Geometry: final body of the model. Coordinates: model frame, mm. Face numbers are marked on the shaded views. A direction names the side the tool comes from. Round coordinates to 2 decimals unless told otherwise and drop trailing zeros. Loops run counter-clockwise (first coordinate to the right, second up) from the corner with the lowest first, then second, coordinate; pieces in that order, holes last. Notation, with made-up numbers: (77.5, -34) - (90.5, -34) arc R13 ccw to (90.5, -30) - close; hole circle Ø1 at (36, -35.75). An arc over 180 degrees is marked (long way). Use CSV: the item, a comma, the result in double quotes.
from build123d import *

# Parameters (mm, degrees)
BASE_EXTRUDE_DEPTH = 19.05


with BuildPart() as part:
    # Sketch1 → Base-Extrude (new body)
    with BuildSketch(Plane.XY):
        with BuildLine():
            Line((-76.2, -6.35), (-196.85, -6.35))
            ThreePointArc((-196.85, -6.35), (-199.09506403, -5.42006403), (-200.025, -3.175))
            Line((-200.025, -3.175), (-200.025, 41.275))
            ThreePointArc((-200.025, 41.275), (-199.09506403, 43.52006403), (-196.85, 44.45))
            Line((-196.85, 44.45), (-76.2, 44.45))
            ThreePointArc((-76.2, 44.45), (-73.95493597, 43.52006403), (-73.025, 41.275))
            Line((-73.025, 41.275), (-73.025, -3.175))
            ThreePointArc((-73.025, -3.175), (-73.95493597, -5.42006403), (-76.2, -6.35))
        make_face()
        with BuildLine():
            Line((-174.625, 11.1125), (-98.425, 11.1125))
            ThreePointArc((-98.425, 11.1125), (-90.4875, 19.05), (-98.425, 26.9875))
            Line((-98.425, 26.9875), (-174.625, 26.9875))
            ThreePointArc((-174.625, 26.9875), (-182.5625, 19.05), (-174.625, 11.1125))
        make_face(mode=Mode.SUBTRACT)
    extrude(amount=BASE_EXTRUDE_DEPTH)


solid = part.part
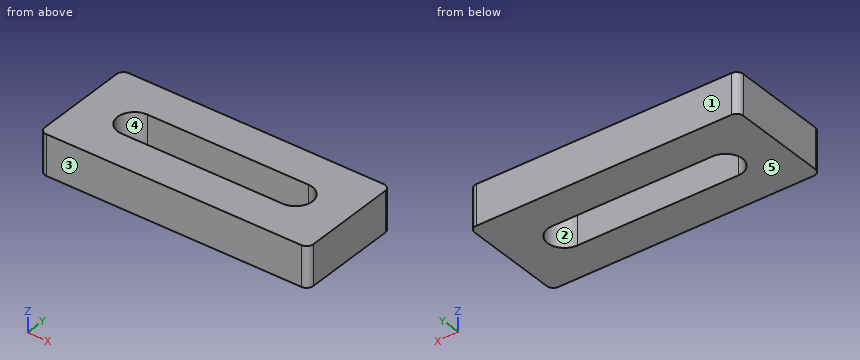
Item 1: Pin query (flat end, axial travel): P1, Ø5, axis at x = -99, y = 16, coming from the -Z side. Return the tip coordinate at first contact, or that it passes through.
Final values:
P1,"passes through"
Item 2: Section B-B on x = -134.5. Return the cut outline in (y, z), plus the area to 3 significant figures.
Final values:
outline,"(-6.35, 0) - (11.11, 0) - (11.11, 19.05) - (-6.35, 19.05) - close; (26.99, 0) - (44.45, 0) - (44.45, 19.05) - (26.99, 19.05) - close"
area,"665 mm²"
Item 3: Mould query, pull axis Y, two halves, no side actions, for the marked faces 3, 4 and 5. Classes: released by +Y, released by -Y, zero draft, split by the parting line, or undercut.
Final values:
face 3,"released by -Y"
face 4,"undercut"
face 5,"zero draft"
Item 4: Reachability of the marked faces 1 and 2 from +Z, -Z, +X, -X, +Y, -Y: full face, straight path, thin tool, end or side. Return the list, or none.
Final values:
face 1,"+Z, -Z, +X, -X, +Y"
face 2,"+Z, -Z"
Item 5: Material intervals for line 1 (Y direction, x = -137, z = 8.75); line 2 (X direction, y = 18, z = 8.5) (3 decimals); line 3 (Y direction, x = -92.5, z = 14.25), sorted ascending.
Final values:
line 1,"y = -6.35 to 11.11, 26.99 to 44.45"
line 2,"x = -200.025 to -182.493, -90.557 to -73.025"
line 3,"y = -6.35 to 13.77, 24.33 to 44.45"
